```python
from build123d import *

# Parameters (mm, degrees)
SKETCH1_R               = 15.875
SKETCH1_R_2             = 4.7625
SKETCH1_R_3             = 12.7
BOSS_EXTRUDE1_DEPTH     = 12.7
SKETCH2_R               = 15.875
SKETCH2_R_2             = 4.7625
SKETCH2_R_3             = 12.7
BOSS_EXTRUDE2_DEPTH     = 12.7
SWEEP_THIN1_PROFILE_R   = 15.875
SWEEP_THIN1_PROFILE_R_2 = 12.7
SWEEP_THIN2_PROFILE_R   = 15.875
SWEEP_THIN2_PROFILE_R_2 = 12.7


with BuildPart() as part:
    # Sketch1 → Boss-Extrude1 (new body)
    # profile 1 of 2: a face of its own
    with BuildSketch(Plane(origin=(0, 0, 0), x_dir=(1, 0, 0), z_dir=(0, 1, 0))):
        with BuildLine():
            Line((-20.953930949, 7.408333333), (-8.980256121, 41.275))
            ThreePointArc((-8.980256121, 41.275), (0, 47.625), (8.980256121, 41.275))
            Line((8.980256121, 41.275), (20.953930949, 7.408333333))
            ThreePointArc((20.953930949, 7.408333333), (22.225, 0), (20.953930949, -7.408333333))
            Line((20.953930949, -7.408333333), (8.980256121, -41.275))
            ThreePointArc((8.980256121, -41.275), (0, -47.625), (-8.980256121, -41.275))
            Line((-8.980256121, -41.275), (-20.953930949, -7.408333333))
            ThreePointArc((-20.953930949, -7.408333333), (-22.225, 0), (-20.953930949, 7.408333333))
        make_face()
        Circle(SKETCH1_R, mode=Mode.SUBTRACT)
        with Locations(Location((0, 38.1, 0), (0, 0, 270))):
            Circle(SKETCH1_R_2, mode=Mode.SUBTRACT)
        with Locations(Location((0, -38.1, 0), (0, 0, 270))):
            Circle(SKETCH1_R_2, mode=Mode.SUBTRACT)
    # profile 2 of 2: a face of its own
    with BuildSketch(Plane(origin=(0, 0, 0), x_dir=(1, 0, 0), z_dir=(0, 1, 0))):
        Circle(SKETCH1_R)
        with Locations(Location((0, 0, 0), (0, 0, 270))):
            Circle(SKETCH1_R_3, mode=Mode.SUBTRACT)
    extrude(amount=-BOSS_EXTRUDE1_DEPTH)

    # Sweep-Thin1: sweep along a path in Sketch3
    with BuildLine(Plane.XY) as sweep_thin1_path:
        ThreePointArc((0, 0), (14.878975516, 35.921024484), (50.8, 50.8))
    # Sweep-Thin1 profile (on start of the path) → Sweep-Thin1 (sweep)
    with BuildSketch(Plane(origin=(0, 0, 0), x_dir=(1, 0, 0), z_dir=(0, 1, 0))):
        Circle(SWEEP_THIN1_PROFILE_R)
        Circle(SWEEP_THIN1_PROFILE_R_2, mode=Mode.SUBTRACT)
    sweep(path=sweep_thin1_path.line)



with BuildPart() as body_2:
    # Sketch2 → Boss-Extrude2 (new body)
    # profile 1 of 2: a face of its own
    with BuildSketch(Plane(origin=(0, 101.6, 0), x_dir=(1, 0, 0), z_dir=(0, 1, 0))):
        with BuildLine():
            Line((80.646069051, 7.408333333), (92.619743879, 41.275))
            ThreePointArc((92.619743879, 41.275), (101.6, 47.625), (110.580256121, 41.275))
            Line((110.580256121, 41.275), (122.553930949, 7.408333333))
            ThreePointArc((122.553930949, 7.408333333), (123.825, 0), (122.553930949, -7.408333333))
            Line((122.553930949, -7.408333333), (110.580256121, -41.275))
            ThreePointArc((110.580256121, -41.275), (101.6, -47.625), (92.619743879, -41.275))
            Line((92.619743879, -41.275), (80.646069051, -7.408333333))
            ThreePointArc((80.646069051, -7.408333333), (79.375, 0), (80.646069051, 7.408333333))
        make_face()
        with Locations((101.6, 0)):
            Circle(SKETCH2_R, mode=Mode.SUBTRACT)
        with Locations(Location((101.6, 38.1, 0), (0, 0, 270))):
            Circle(SKETCH2_R_2, mode=Mode.SUBTRACT)
        with Locations(Location((101.6, -38.1, 0), (0, 0, 270))):
            Circle(SKETCH2_R_2, mode=Mode.SUBTRACT)
    # profile 2 of 2: a face of its own
    with BuildSketch(Plane(origin=(0, 101.6, 0), x_dir=(1, 0, 0), z_dir=(0, 1, 0))):
        with Locations((101.6, 0)):
            Circle(SKETCH2_R)
        with Locations(Location((101.6, 0, 0), (0, 0, 270))):
            Circle(SKETCH2_R_3, mode=Mode.SUBTRACT)
    extrude(amount=BOSS_EXTRUDE2_DEPTH)


with BuildPart() as part_1:
    add(part.part)

    add(body_2.part)  # Sweep-Thin2 merges body 2
    # Sweep-Thin2: sweep along a path in Sketch25
    with BuildLine(Plane.XY) as sweep_thin2_path:
        ThreePointArc((101.6, 101.6), (86.721024484, 65.678975516), (50.8, 50.8))
    # Sweep-Thin2 profile (on start of the path) → Sweep-Thin2 (sweep)
    with BuildSketch(Plane(origin=(101.6, 101.6, 0), x_dir=(-1, 0, 0), z_dir=(0, -1, 0))):
        Circle(SWEEP_THIN2_PROFILE_R)
        Circle(SWEEP_THIN2_PROFILE_R_2, mode=Mode.SUBTRACT)
    sweep(path=sweep_thin2_path.line)


solid = part_1.part
```
Input: part model. Units: mm. Frame: model coordinates. A direction names the side the tool comes from. Give positions to 0.01 mm unless a question says otherwise; leave off trailing zeros. Order: outer loops, then holes, each group sorted by start corner. A loop starts at its lowest first (then second) coordinate and runs counter-clockwise, first axis right, second up. Notation, with made-up numbers: M -30.75,37 L -26.75,37 A25 ccw -26.75,50 Z; hole C 89,23 d7. An arc over 180 degrees is marked long. One line per question, with ' | ' between items. Start each with the question number.
1. First-contact query: pin 1 Ø5 at (y, z) = (27, 11.5) entering from +X; pin 2 Ø12.5 at (x, z) = (0, -38.1) entering from +Y; pin 3 Ø20.5 at (x, z) = (0, 0) entering from +Y; pin 4 Ø8.5 at (x, z) = (0, 38.1) entering from +Y. Flat tips, straight axial feed; report the tip coordinate or a pass-through.
2. Pull-direction query (Z, two-part tool) for faces 1 (the face through (-0.164, -6.261, -47.624)), 2 (the face through (1.431, -6.261, 42.643)), 3 (the face through (-22.225, -6.261, 0.106)), 4 (the face through (0.164, -6.261, 47.624)); classes: released by +Z, released by -Z, zero draft, split by the parting line, or undercut.
3. Section query C-C (z = 0). Return the cut outline in (x, y) (3 decimals), and give its area (3 significant figures).
4. Material intervals for probe 1 along X at (y, z) = (-6.5, 0) (3 decimals); probe 2 along X at (y, z) = (106, 41); probe 3 along Y at (x, z) = (44, 3.5), sorted ascending. Write a range as [from, to].
5. Access query for faces 5 (the face through (79.375, 107.861, 0.106)), 6 (the face through (86.717, 107.861, 24.579)), 7 (the face through (22.225, -6.261, -0.106)), 8 (the face through (86.549, 107.861, -24.105)). Directions: +Z, -Z, +X, -X, +Y, -Y. A direction counts if a zero-diameter tool reaches every point of the face in a straight line with its end or side. Return the directions, or none.
6. Section query A-A (z = 39). Return the cut outline in (x, y).
7. Section query B-B (y = -4). Count the separate pieces of the cut face and the enclosed holes in it, and give its area (3 significant figures).
Here are the results:
1) pin 1: x = 25.58 | pin 2: y = 0 | pin 3: y = 52.93 | pin 4: through
2) face 1: released by -Z | face 2: undercut | face 3: split by the parting line | face 4: released by +Z
3) outline: M -22.225,-12.7 L -12.7,-12.7 L -12.7,0 A63.5 cw 50.8,63.5 A38.1 ccw 88.9,101.6 L 88.9,114.3 L 79.375,114.3 L 79.375,101.6 L 85.725,101.6 A34.925 cw 50.8,66.675 A66.675 ccw -15.875,0 L -22.225,0 Z; M 12.7,-12.7 L 22.225,-12.7 L 22.225,0 L 15.875,0 A34.925 cw 50.8,34.925 A66.675 ccw 117.475,101.6 L 123.825,101.6 L 123.825,114.3 L 114.3,114.3 L 114.3,101.6 A63.5 cw 50.8,38.1 A38.1 ccw 12.7,0 Z | area: 1,500 mm²
4) probe 1: [-22.225, -12.7], [12.7, 22.225] | probe 2: [92.52, 97.82], [105.38, 110.68] | probe 3: [34.65, 37.99], [62.64, 65.93]
5) face 5: -X, +Y | face 6: +Z, -X, +Y | face 7: +X, -Y | face 8: -Z, -X, +Y
6) outline: M -9.78,-12.7 L -4.68,-12.7 L -4.68,0 L -9.78,0 Z; M 4.68,-12.7 L 9.78,-12.7 L 9.78,0 L 4.68,0 Z; M 91.82,101.6 L 96.92,101.6 L 96.92,114.3 L 91.82,114.3 Z; M 106.28,101.6 L 111.38,101.6 L 111.38,114.3 L 106.28,114.3 Z
7) separate pieces: 1 | enclosed holes: 3 | area: 2,190 mm²
